Read the model definition and answer for the solid it produces. Units are mm, in the model's axes. A direction names the side the tool comes from. Coordinates: 2 decimals unless noted, no trailing zeros. Order: outer loops, then holes, each group sorted by start corner. A loop starts at its lowest first (then second) coordinate and runs counter-clockwise, first axis right, second up. Notation, with made-up numbers: (45, 86) -> (74, 86) arc R21 cw to (74, 110) -> close; hole circle Ø5 at (-7.5, 48.25). An arc over 180 degrees is marked (long way). Answer as a JSON object with one key per item and string values. Group by question number.
1) A tool of negligible diameter and unlimited length cuts with its end or side. For faces 5 (the flat face through (1.324, 1.47, -17.003)), 6 (the cylindrical face through (4.31, 2.52, -8.87)), from which of +Z, -Z, +X, -X, +Y, -Y can it reach the whole face along a straight path? Write none if from no direction.
2) Given pin 1 (1.1 mm diameter, centred on y = 1.5, z = -11, fed in from -X); pin 2 (8.5 mm diameter, centred on x = 10.5, z = -11.5, fed in from +Y), each flat-ended and moving along its own axis, determine where each tip first touches the part or whether it passes through.
3) Section D-D on y = 1.85 is taken. Determine the outline of the cut face in (x, z).
4) Section C-C on z = -10.75 is taken. Determine the outline of the cut face in (x, y) (3 decimals).
5) Section A-A on y = 3.45 is taken. Determine the outline of the cut face in (x, z), and give its area (3 significant figures).
6) Determine the mould class of faces 1 (the flat face through (1.271, 1.527, -5.946)), 2 (the flat face through (3, 1, -12)), 3 (the flat face through (8, 2, 0)), 4 (the flat face through (0, 2, -2)) for opening direction Z: released by +Z, released by -Z, zero draft, split by the parting line, or undercut.
7) Consider L1, parallel to X at y = 2.05, z = -14.5; L2, parallel to X at y = 3.2, z = -9.75; L3, parallel to X at y = 3.3, z = -2.5. Determine where each line is inside the solid, lowest interval first.
8) Section B-B on x = 10.5 is taken. Determine the outline of the cut face in (y, z), and give its area (3 significant figures).
from build123d import *

# Parameters (mm, degrees)
BOSS_EXTRUDE1_DEPTH      = 5
BOSS_EXTRUDE1_DEPTH_BACK = 0.0001
SKETCH1_R                = 2.6
SKETCH2_R                = 3.075
CUT_EXTRUDE1_DEPTH       = 24.958297101
FILLET1_R                = 2.5
SKETCH3_W                = 0.717338371
SKETCH3_H                = 1
CUT_EXTRUDE2_DEPTH       = 24.958297101
SKETCH4_W                = 0.2
SKETCH4_H                = 18
CUT_EXTRUDE3_DEPTH       = 24.958317971


with BuildPart() as part:
    # Sketch1 → Boss-Extrude1 (new, two sides: drawn at the far end of the back side and taken through both)
    with BuildSketch(Plane(origin=(0, 0, 0), x_dir=(1, 0, 0), z_dir=(0, 1, 0)).offset(-BOSS_EXTRUDE1_DEPTH_BACK)):
        Polygon((0, 18), (2.8, 15.304069131), (2.8, 7.695628029), (0, 5), (0, 0), (15, 0), (15, 18), align=None)
        with Locations(Location((10.5, 11.499529694, 0), (0, 0, 270))):
            Circle(SKETCH1_R, mode=Mode.SUBTRACT)
    extrude(amount=BOSS_EXTRUDE1_DEPTH + BOSS_EXTRUDE1_DEPTH_BACK)

    # Sketch2 → Cut-Extrude1 (cut, through all)
    with BuildSketch(Plane.XY):
        with Locations((3, 5.3)):
            Circle(SKETCH2_R)
    extrude(amount=-CUT_EXTRUDE1_DEPTH, mode=Mode.SUBTRACT)

    # Fillet1
    fillet1_edges = [part.edges().sort_by_distance(p)[0] for p in [
        (15, 2.49995, 0),
    ]]
    fillet(fillet1_edges, radius=FILLET1_R)

    # Sketch3 → Cut-Extrude2 (cut, through all)
    with BuildSketch(Plane.XY):
        with Locations((0.358669186, 4.5)):
            Rectangle(SKETCH3_W, SKETCH3_H)
    extrude(amount=-CUT_EXTRUDE2_DEPTH, mode=Mode.SUBTRACT)

    # Sketch4 → Cut-Extrude3 (cut, through all)
    with BuildSketch(Plane.XZ.offset(0.0001)):
        Polygon((0.138710494, -4.855918777), (-0.903561635, -4.855918777), (-0.903561635, -18.144073437), (0.138718581, -18.144073437), (3, -15.389138829), (3, -7.610551703), align=None)
        with Locations((14.9, -9)):
            Rectangle(SKETCH4_W, SKETCH4_H)
    extrude(amount=-CUT_EXTRUDE3_DEPTH, mode=Mode.SUBTRACT)


solid = part.part
Worked answers:
{
 "1": {"face 5": "-X, +Y, -Y", "face 6": "+Z, -Z, +Y"},
 "2": {"pin 1": "stops at x = 3", "pin 2": "stops at y = 5"},
 "3": {"outline": "(0, -4.86) -> (0.14, -4.86) -> (3, -7.61) -> (3, -15.39) -> (0.29, -18) -> (14.8, -18) -> (14.8, -1.52) arc R2.5 ccw to (12.5, 0) -> (0, 0) -> close; hole circle Ø5.2 at (10.5, -11.5)"},
 "4": {"outline": "(3, 0) -> (8.01, 0) -> (8.01, 5) -> (6.06, 5) arc R3.075 cw to (3, 2.225) -> close; (12.99, 0) -> (14.8, 0) -> (14.8, 5) -> (12.99, 5) -> close"},
 "5": {"outline": "(0, -4.86) -> (0.14, -4.86) -> (0.54, -5.25) -> (0.54, 0) -> (0, 0) -> close; (0.29, -18) -> (0.54, -18) -> (0.54, -17.75) -> close; (5.46, -18) -> (14.8, -18) -> (14.8, -1.52) arc R2.5 ccw to (12.5, 0) -> (5.46, 0) -> close; hole circle Ø5.2 at (10.5, -11.5)", "area": "149 mm²"},
 "6": {"face 1": "undercut", "face 2": "undercut", "face 3": "released by +Z", "face 4": "zero draft"},
 "7": {"L1": "x = 3 to 14.8", "L2": "x = 5.25 to 8.58, 12.42 to 14.8", "L3": "x = 0 to 0.66, 5.34 to 14.8"},
 "8": {"outline": "(0, -18) -> (5, -18) -> (5, -14.1) -> (0, -14.1) -> close; (0, -8.9) -> (5, -8.9) -> (5, 0) -> (0, 0) -> close", "area": "64.0 mm²"}
}
